Part model, mm, in its own coordinate system. Coordinates: 2 decimals unless noted, no trailing zeros. Loops run counter-clockwise (first coordinate to the right, second up) from the corner with the lowest first, then second, coordinate; pieces in that order, holes last. Notation, with made-up numbers: (-32.75, -21) - (-12.75, -21) arc R16 ccw to (-12.75, -13) - close; hole circle Ø7 at (-24, 25.5). An arc over 180 degrees is marked (long way). Use a Markdown table: item, result. Add a question column.
1) Band-saw the part on A-A (x = 375). Give the cut face in (y, z), plus the area to 3 significant figures.
2) Band-saw the part on C-C (x = 21.5). Give the cut face in (y, z).
3) Drop flat-ended pins along their axis: P1, Ø0.6, axis at y = 1, z = 17.5, coming from the -X side; P2, Ø0.6, axis at x = 731.5, y = 1, coming from the +Z side. Give the stop position or say it passes through.
4) Probe probe 1 along Z at (x, y) = (209.5, 0.2); probe 2 along Z at (x, y) = (368, 0.35). List the from-to ranges inside material, lowest first. Write a range as [from, to].
5) Band-saw the part on B-B (y = 1.6). Give the number of separate pieces and of enclosed holes in the cut face, plus the area to 3 significant figures.
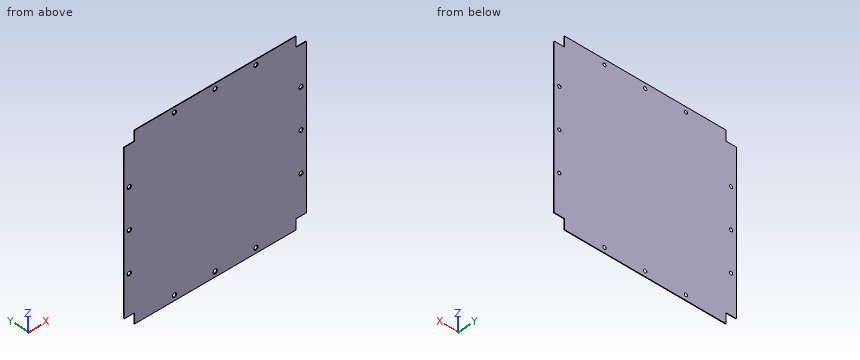
from build123d import *

# Parameters (mm, degrees)
BOSS_EXTRUDE2_DEPTH                            = 2
CSK_FOR_M8_FLAT_HEAD_MACHINE_SCREW2_AT_2_COUNT = 2
CSK_FOR_M8_FLAT_HEAD_MACHINE_SCREW2_AT_2_PITCH = 167.5
CSK_FOR_M8_FLAT_HEAD_MACHINE_SCREW2_AT_3_COUNT = 2
CSK_FOR_M8_FLAT_HEAD_MACHINE_SCREW2_AT_3_PITCH = 167.5
CSK_FOR_M8_FLAT_HEAD_MACHINE_SCREW2_AT_4_COUNT = 2
CSK_FOR_M8_FLAT_HEAD_MACHINE_SCREW2_AT_4_PITCH = 399.447430834
CSK_FOR_M8_FLAT_HEAD_MACHINE_SCREW2_AT_5_COUNT = 2
CSK_FOR_M8_FLAT_HEAD_MACHINE_SCREW2_AT_5_PITCH = 629.605630534


with BuildPart() as part:
    # Sketch3 → Boss-Extrude2 (new body)
    with BuildSketch(Plane(origin=(0, 0, 0), x_dir=(1, 0, 0), z_dir=(0, 1, 0))):
        Polygon((750, -707), (750, -43), (707, -43), (707, 0), (43, 0), (43, -43), (0, -43), (0, -707), (43, -707), (43, -750), (707, -750), (707, -707), align=None)
    extrude(amount=BOSS_EXTRUDE2_DEPTH)

    # Sketch9 → CSK for M8 Flat Head Machine Screw1 (revolve, cut)
    with BuildSketch(Plane(origin=(21.5, 0, 375), x_dir=(0, 0, -1), z_dir=(1, 0, 0))):
        Polygon((0, 0), (0, 2), (4.5, 2), (4.5, 4.15), (8.65, 0), align=None)
    csk_for_m8_flat_head_machine_screw1 = revolve(axis=Axis((21.5, -6.35, 375), (0, 1, 0)), mode=Mode.SUBTRACT)

    # Sketch12 → CSK for M8 Flat Head Machine Screw2 (revolve, cut)
    with BuildSketch(Plane(origin=(375, 0, 728.5), x_dir=(0, 0, -1), z_dir=(1, 0, 0))):
        Polygon((0, 0), (0, 2), (4.5, 2), (4.5, 4.15), (8.65, 0), align=None)
    csk_for_m8_flat_head_machine_screw2 = revolve(axis=Axis((375, -6.35, 728.5), (0, 1, 0)), mode=Mode.SUBTRACT)

    # CSK for M8 Flat Head Machine Screw2 at 2: CSK for M8 Flat Head Machine Screw2 ×2
    with Locations(*[(i * CSK_FOR_M8_FLAT_HEAD_MACHINE_SCREW2_AT_2_PITCH, 0, 0) for i in range(1, CSK_FOR_M8_FLAT_HEAD_MACHINE_SCREW2_AT_2_COUNT)]):
        add(csk_for_m8_flat_head_machine_screw2, mode=Mode.SUBTRACT)

    # CSK for M8 Flat Head Machine Screw2 at 3: CSK for M8 Flat Head Machine Screw2 ×2
    with Locations(*[(-i * CSK_FOR_M8_FLAT_HEAD_MACHINE_SCREW2_AT_3_PITCH, 0, 0) for i in range(1, CSK_FOR_M8_FLAT_HEAD_MACHINE_SCREW2_AT_3_COUNT)]):
        add(csk_for_m8_flat_head_machine_screw2, mode=Mode.SUBTRACT)

    # CSK for M8 Flat Head Machine Screw2 at 4: CSK for M8 Flat Head Machine Screw2 ×2
    with Locations(*[Vector(-0.884972521, 0, -0.46564325) * (i * CSK_FOR_M8_FLAT_HEAD_MACHINE_SCREW2_AT_4_PITCH) for i in range(1, CSK_FOR_M8_FLAT_HEAD_MACHINE_SCREW2_AT_4_COUNT)]):
        add(csk_for_m8_flat_head_machine_screw2, mode=Mode.SUBTRACT)

    # CSK for M8 Flat Head Machine Screw2 at 5: CSK for M8 Flat Head Machine Screw2 ×2
    with Locations(*[Vector(-0.561462577, 0, -0.827502129) * (i * CSK_FOR_M8_FLAT_HEAD_MACHINE_SCREW2_AT_5_PITCH) for i in range(1, CSK_FOR_M8_FLAT_HEAD_MACHINE_SCREW2_AT_5_COUNT)]):
        add(csk_for_m8_flat_head_machine_screw2, mode=Mode.SUBTRACT)

    # Mirror1: CSK for M8 Flat Head Machine Screw1, CSK for M8 Flat Head Machine Screw2 across plane
    add(csk_for_m8_flat_head_machine_screw1.mirror(Plane.ZY.offset(-375)), mode=Mode.SUBTRACT)
    add(csk_for_m8_flat_head_machine_screw2.mirror(Plane.ZY.offset(-375)), mode=Mode.SUBTRACT)

    # Mirror1 copy 1 sketch → Mirror1 copy 1 (revolve, cut)
    with BuildSketch(Plane(origin=(207.5, 0, 728.5), x_dir=(0, 0, -1), z_dir=(-1, 0, 0))):
        Polygon((0, 0), (0, -2), (4.5, -2), (4.5, -4.15), (8.65, 0), align=None)
    revolve(axis=Axis((207.5, -6.35, 728.5), (0, -1, 0)), mode=Mode.SUBTRACT)

    # Mirror1 copy 2 sketch → Mirror1 copy 2 (revolve, cut)
    with BuildSketch(Plane(origin=(542.5, 0, 728.5), x_dir=(0, 0, -1), z_dir=(-1, 0, 0))):
        Polygon((0, 0), (0, -2), (4.5, -2), (4.5, -4.15), (8.65, 0), align=None)
    revolve(axis=Axis((542.5, -6.35, 728.5), (0, -1, 0)), mode=Mode.SUBTRACT)

    # Mirror1 copy 3 sketch → Mirror1 copy 3 (revolve, cut)
    with BuildSketch(Plane(origin=(728.5, 0, 542.5), x_dir=(0, 0, -1), z_dir=(-1, 0, 0))):
        Polygon((0, 0), (0, -2), (4.5, -2), (4.5, -4.15), (8.65, 0), align=None)
    revolve(axis=Axis((728.5, -6.35, 542.5), (0, -1, 0)), mode=Mode.SUBTRACT)

    # Mirror1 copy 4 sketch → Mirror1 copy 4 (revolve, cut)
    with BuildSketch(Plane(origin=(728.5, 0, 207.5), x_dir=(0, 0, -1), z_dir=(-1, 0, 0))):
        Polygon((0, 0), (0, -2), (4.5, -2), (4.5, -4.15), (8.65, 0), align=None)
    revolve(axis=Axis((728.5, -6.35, 207.5), (0, -1, 0)), mode=Mode.SUBTRACT)

    # Mirror2: CSK for M8 Flat Head Machine Screw2 across plane
    add(csk_for_m8_flat_head_machine_screw2.mirror(Plane.XY.offset(375)), mode=Mode.SUBTRACT)

    # Mirror2 copy 1 sketch → Mirror2 copy 1 (revolve, cut)
    with BuildSketch(Plane(origin=(542.5, 0, 21.5), x_dir=(0, 0, 1), z_dir=(1, 0, 0))):
        Polygon((0, 0), (0, -2), (4.5, -2), (4.5, -4.15), (8.65, 0), align=None)
    revolve(axis=Axis((542.5, -6.35, 21.5), (0, -1, 0)), mode=Mode.SUBTRACT)

    # Mirror2 copy 2 sketch → Mirror2 copy 2 (revolve, cut)
    with BuildSketch(Plane(origin=(207.5, 0, 21.5), x_dir=(0, 0, 1), z_dir=(1, 0, 0))):
        Polygon((0, 0), (0, -2), (4.5, -2), (4.5, -4.15), (8.65, 0), align=None)
    revolve(axis=Axis((207.5, -6.35, 21.5), (0, -1, 0)), mode=Mode.SUBTRACT)

    # Mirror2 copy 3 sketch → Mirror2 copy 3 (revolve, cut)
    with BuildSketch(Plane(origin=(21.5, 0, 207.5), x_dir=(0, 0, 1), z_dir=(1, 0, 0))):
        Polygon((0, 0), (0, -2), (4.5, -2), (4.5, -4.15), (8.65, 0), align=None)
    revolve(axis=Axis((21.5, -6.35, 207.5), (0, -1, 0)), mode=Mode.SUBTRACT)

    # Mirror2 copy 4 sketch → Mirror2 copy 4 (revolve, cut)
    with BuildSketch(Plane(origin=(21.5, 0, 542.5), x_dir=(0, 0, 1), z_dir=(1, 0, 0))):
        Polygon((0, 0), (0, -2), (4.5, -2), (4.5, -4.15), (8.65, 0), align=None)
    revolve(axis=Axis((21.5, -6.35, 542.5), (0, -1, 0)), mode=Mode.SUBTRACT)


solid = part.part
Answer block:
| question | item | result |
|---|---|---|
| 1 | outline | (0, 0) - (2, 0) - (2, 14.85) - (0, 12.85) - close; (0, 30.15) - (2, 28.15) - (2, 721.85) - (0, 719.85) - close; (0, 737.15) - (2, 735.15) - (2, 750) - (0, 750) - close |
| 1 | area | 1,440 mm2 |
| 2 | outline | (0, 43) - (2, 43) - (2, 200.85) - (0, 198.85) - close; (0, 216.15) - (2, 214.15) - (2, 368.35) - (0, 366.35) - close; (0, 383.65) - (2, 381.65) - (2, 535.85) - (0, 533.85) - close; (0, 551.15) - (2, 549.15) - (2, 707) - (0, 707) - close |
| 3 | P1 | x = 43 |
| 3 | P2 | z = 707 |
| 4 | probe 1 | [0, 13.29], [29.71, 720.29], [736.71, 750] |
| 4 | probe 2 | [0, 17.04], [25.96, 724.04], [732.96, 750] |
| 5 | separate pieces | 1 |
| 5 | enclosed holes | 12 |
| 5 | area | 553,000 mm2 |
